Check sheet for the modelled part. Datum: model origin and axes. Units: mm. Give positions to 0.01 mm unless a question says otherwise; leave off trailing zeros. Order: outer loops, then holes, each group sorted by start corner. A loop starts at its lowest first (then second) coordinate and runs counter-clockwise, first axis right, second up. Notation, with made-up numbers: M 14.25,25.5 L 63.25,25.5 A26 cw 63.25,60.5 Z; hole C 55.5,-23.75 d8. An arc over 180 degrees is marked long. Answer in a Markdown table with one row per item. Add a question column.
from build123d import *

# Parameters (mm, degrees)
F0_W     = 450
F0_H     = 1000
F1_DEPTH = 82
F2_W     = 18
F2_H     = 18
F3_DEPTH = 25
F4_SIZE  = 1


with BuildPart() as f1:
    # F0 (on Front) → F1 (new body)
    with BuildSketch(Plane.XZ):
        Rectangle(F0_W, F0_H)
        Polygon((-207, 482), (207, 482), (207, -482), (9, -482), (9, -182), (-9, -182), (-9, -482), (-207, -482), align=None, mode=Mode.SUBTRACT)
    extrude(amount=F1_DEPTH)

    # F2 (on face) → F3 (cut)
    with BuildSketch(Plane.YZ.offset(9)):
        with Locations((-9, -191)):
            Rectangle(F2_W, F2_H)
    extrude(amount=-F3_DEPTH, mode=Mode.SUBTRACT)

    # F4
    f4_edges = [f1.edges().sort_by_distance(p)[0] for p in [
        (0, -82, 500),
        (0, 0, -500),
        (-225, -41, 500),
        (225, -41, 500),
        (225, -41, -500),
        (9, -41, -482),
        (-207, -41, -482),
        (0, 0, 500),
        (9, -82, -332),
        (225, 0, 0),
        (-108, 0, -482),
        (225, -82, 0),
        (0, 0, 482),
        (108, 0, -482),
        (207, 0, 0),
        (9, -9, -200),
        (0, -82, -500),
        (-225, -41, -500),
        (207, -41, 482),
        (-207, -41, 482),
        (207, -41, -482),
        (-9, -41, -482),
        (0, 0, -200),
        (0, -18, -182),
        (-9, -82, -332),
        (0, -82, -182),
        (-225, 0, 0),
        (-225, -82, 0),
        (-108, -82, -482),
        (0, -18, -200),
        (0, -82, 482),
        (108, -82, -482),
        (207, -82, 0),
        (-207, 0, 0),
        (-207, -82, 0),
        (9, -18, -191),
        (-9, -9, -200),
        (-9, -18, -191),
        (-9, 0, -341),
        (9, 0, -341),
        (9, -50, -182),
        (-9, -50, -182),
    ]]
    chamfer(f4_edges, length=F4_SIZE)


solid = f1.part
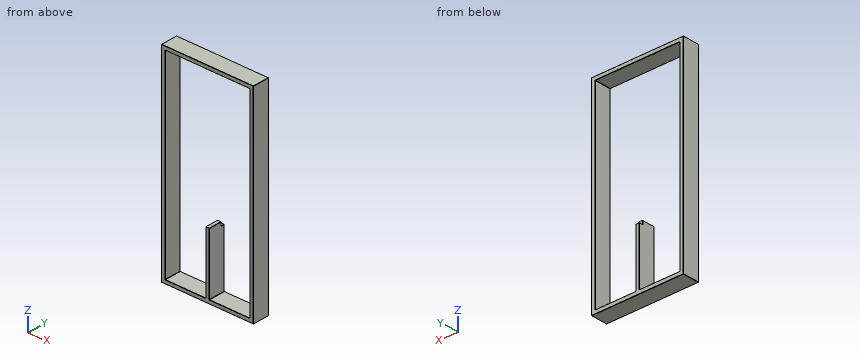
Q1. Cross-section at D-D (z = -227.5). Record the boundary of the cut face in (x, y), and give its area (3 significant figures).
Q2. Go/stop test with a flat-tipped pin: pin 1 (17.5 mm diameter, centred on x = 2, z = -188, fed in from +Y). Record where the tip stops, or that it passes through.
Q3. Cross-section at B-B (z = 237). Record the boundary of the cut face in (x, y).
Q4. Thickness scan on probe 1 along X at (y, z) = (-4, -384); probe 2 along Z at (x, y) = (-154.5, -55); probe 3 along X at (y, z) = (-29.5, 212). Record the ranges inside material, lowest first.
Q5. Cross-section at C-C (y = -43). Record the boundary of the cut face in (x, z), and give its area (3 significant figures).
Q6. Cross-section at A-A (x = 99). Record the boundary of the cut face in (y, z), and give its area (3 significant figures).
Values follow:
| question | item | result |
|---|---|---|
| 1 | outline | M -225,-81 L -224,-82 L -208,-82 L -207,-81 L -207,-1 L -208,0 L -224,0 L -225,-1 Z; M -9,-81 L -8,-82 L 8,-82 L 9,-81 L 9,-1 L 8,0 L -8,0 L -9,-1 Z; M 207,-81 L 208,-82 L 224,-82 L 225,-81 L 225,-1 L 224,0 L 208,0 L 207,-1 Z |
| 1 | area | 4,420 mm² |
| 2 | pin 1 | y = -18 |
| 3 | outline | M -225,-81 L -224,-82 L -208,-82 L -207,-81 L -207,-1 L -208,0 L -224,0 L -225,-1 Z; M 207,-81 L 208,-82 L 224,-82 L 225,-81 L 225,-1 L 224,0 L 208,0 L 207,-1 Z |
| 4 | probe 1 | -225 to -207, -9 to 9, 207 to 225 |
| 4 | probe 2 | -500 to -482, 482 to 500 |
| 4 | probe 3 | -225 to -207, 207 to 225 |
| 5 | outline | M -225,-499 L -224,-500 L 224,-500 L 225,-499 L 225,499 L 224,500 L -224,500 L -225,499 Z; hole M -207,-481 L -206,-482 L -10,-482 L -9,-481 L -9,-183 L -8,-182 L 8,-182 L 9,-183 L 9,-481 L 10,-482 L 206,-482 L 207,-481 L 207,481 L 206,482 L -206,482 L -207,481 Z |
| 5 | area | 56,300 mm² |
| 6 | outline | M -82,-499 L -81,-500 L -1,-500 L 0,-499 L 0,-483 L -1,-482 L -81,-482 L -82,-483 Z; M -82,483 L -81,482 L -1,482 L 0,483 L 0,499 L -1,500 L -81,500 L -82,499 Z |
| 6 | area | 2,950 mm² |
